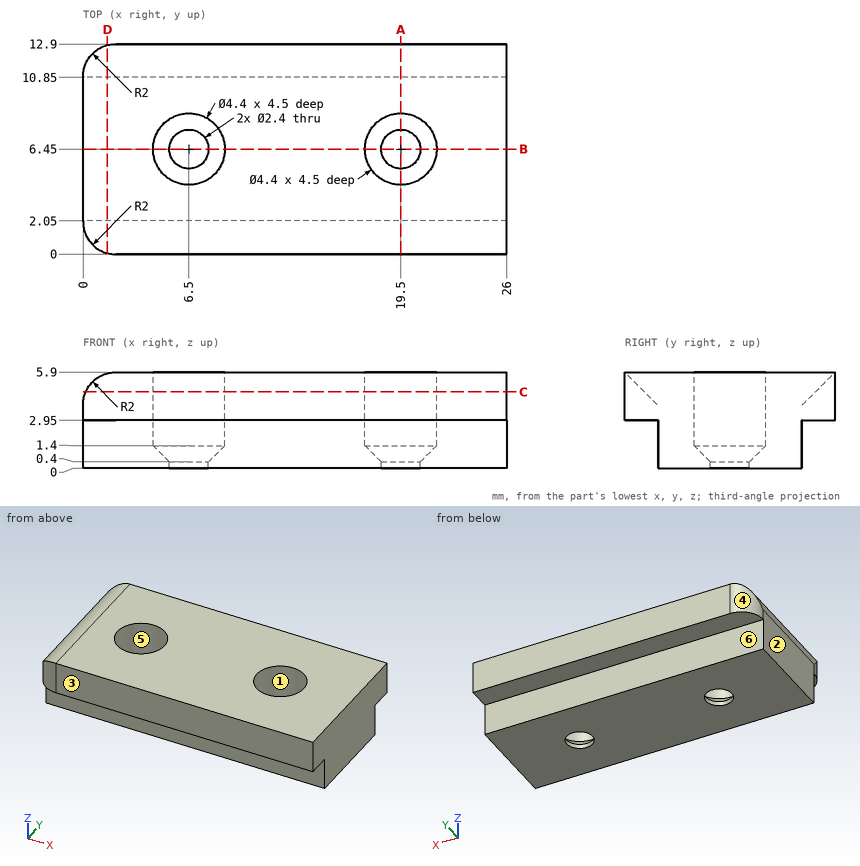
Geometry: see drawing. Coordinates: mm, zero at the bounding-box minimum. A direction names the side the tool comes from. Round coordinates to 2 decimals unless told otherwise and drop trailing zeros. Order: outer loops, then holes, each group sorted by start corner. A loop starts at its lowest first (then second) coordinate and runs counter-clockwise, first axis right, second up. Notation, with made-up numbers: (52.25, -14.75) -> (77.25, -14.75) arc R15 cw to (77.25, 6.25) -> close; hole circle Ø10 at (74.5, -6.75). An arc over 180 degrees is marked (long way). Answer as CSV lines item,"result".
Item 1: Pin query (flat end, axial travel): pin 1 Ø0.9 at (x, z) = (17.5, 1) entering from -Y; pin 2 Ø3 at (x, y) = (6.5, 6.45) entering from +Z; pin 3 Ø1 at (x, y) = (7, 8) entering from +Z. Return the tip coordinate at first contact, or that it passes through.
A:
pin 1,"y = 2.05"
pin 2,"z = 0.7"
pin 3,"z = 1.33"
Item 2: Pull-direction query (X, two-part tool) for the marked faces 1, 2 and 3; classes: pulls with the +X half, pulls with the -X half, needs draft (parallel to the pull), parting line crosses it, or undercut.
A:
face 1,"undercut"
face 2,"pulls with the -X half"
face 3,"needs draft"
Item 3: Reachability of the marked faces 4, 5 and 6 from +Z, -Z, +X, -X, +Y, -Y: full face, straight path, thin tool, end or side. Return the list, or none.
A:
face 4,"+Z, -Z, -X, +Y"
face 5,"+Z"
face 6,"-Z, +X, -X, +Y"
Item 4: Line query: L1, parallel to X at y = 6.45, z = 2.75; L2, parallel to Y at x = 19.5, z = 0.35; L3, parallel to X at y = 8, z = 4.45. Output: solid intervals per line, ascending.
A:
L1,"0 to 4.3, 8.7 to 17.3, 21.7 to 26"
L2,"2.05 to 5.25, 7.65 to 10.85"
L3,"0.08 to 4.94, 8.06 to 17.94, 21.06 to 26"
Item 5: Section C-C, the plane z = 4.7. Return loops of the section in (x, y).
A:
outline,"(0.17, 1.2) arc R2 ccw to (2, 0) -> (26, 0) -> (26, 12.9) -> (2, 12.9) arc R2 ccw to (0.17, 11.7) -> close; hole circle Ø4.4 at (6.5, 6.45); hole circle Ø4.4 at (19.5, 6.45)"
Item 6: Section D-D, the plane x = 1.5. Return loops of the section in (y, z).
A:
outline,"(0.06, 2.95) -> (2.05, 2.95) -> (2.05, 0) -> (10.85, 0) -> (10.85, 2.95) -> (12.84, 2.95) -> (12.84, 5.84) -> (0.06, 5.84) -> close"
Item 7: Section A-A, the plane x = 19.5. Return loops of the section in (y, z), plus the area to 3 significant figures.
A:
outline,"(0, 2.95) -> (2.05, 2.95) -> (2.05, 0) -> (5.25, 0) -> (5.25, 0.4) -> (4.25, 1.4) -> (4.25, 5.9) -> (0, 5.9) -> close; (7.65, 0) -> (10.85, 0) -> (10.85, 2.95) -> (12.9, 2.95) -> (12.9, 5.9) -> (8.65, 5.9) -> (8.65, 1.4) -> (7.65, 0.4) -> close"
area,"39.9 mm²"
Item 8: Section B-B, the plane y = 6.45. Return loops of the section in (x, z).
A:
outline,"(0, 0) -> (5.3, 0) -> (5.3, 0.4) -> (4.3, 1.4) -> (4.3, 5.9) -> (2, 5.9) arc R2 ccw to (0, 3.9) -> close; (7.7, 0) -> (18.3, 0) -> (18.3, 0.4) -> (17.3, 1.4) -> (17.3, 5.9) -> (8.7, 5.9) -> (8.7, 1.4) -> (7.7, 0.4) -> close; (20.7, 0) -> (26, 0) -> (26, 5.9) -> (21.7, 5.9) -> (21.7, 1.4) -> (20.7, 0.4) -> close"
